Check sheet for the drawn part. Datum: minimum x, y, z corner. Units: mm. Round coordinates to 2 decimals unless told otherwise and drop trailing zeros. Write each loop counter-clockwise with the first axis right and the second up, starting at its lowest first coordinate (ties: lowest second). Pieces come first, ordered by that corner, then holes. Notation, with made-up numbers: (48, -9.75) - (106, -9.75) arc R24 ccw to (106, 0.25) - close; hole circle Ø8 at (-14, 12). An arc over 180 degrees is marked (long way). Answer as a JSON object with one key per item and string values. Group by question number.
Item 1: Sectioned sample at B-B on z = 164. Record the boundary of the cut face in (x, y).
Item 2: Thickness scan on line 1 (X direction, y = 0.85, z = 164); line 2 (Z direction, x = 65, y = 0.65) (3 decimals); line 3 (Z direction, x = 82, y = 1.25) (3 decimals). Record the ranges inside material, lowest first.
Item 3: Sectioned sample at A-A on x = 65. Record the boundary of the cut face in (y, z) (3 decimals).
Item 4: Gauge pin test, flat ends, axial feed: P1, Ø2.5, axis at x = 65, z = 164, coming from the +Y side; P2, Ø1.2, axis at y = 3, z = 2, coming from the +X side. Record the tip position at first contact, or that the pin passes through.
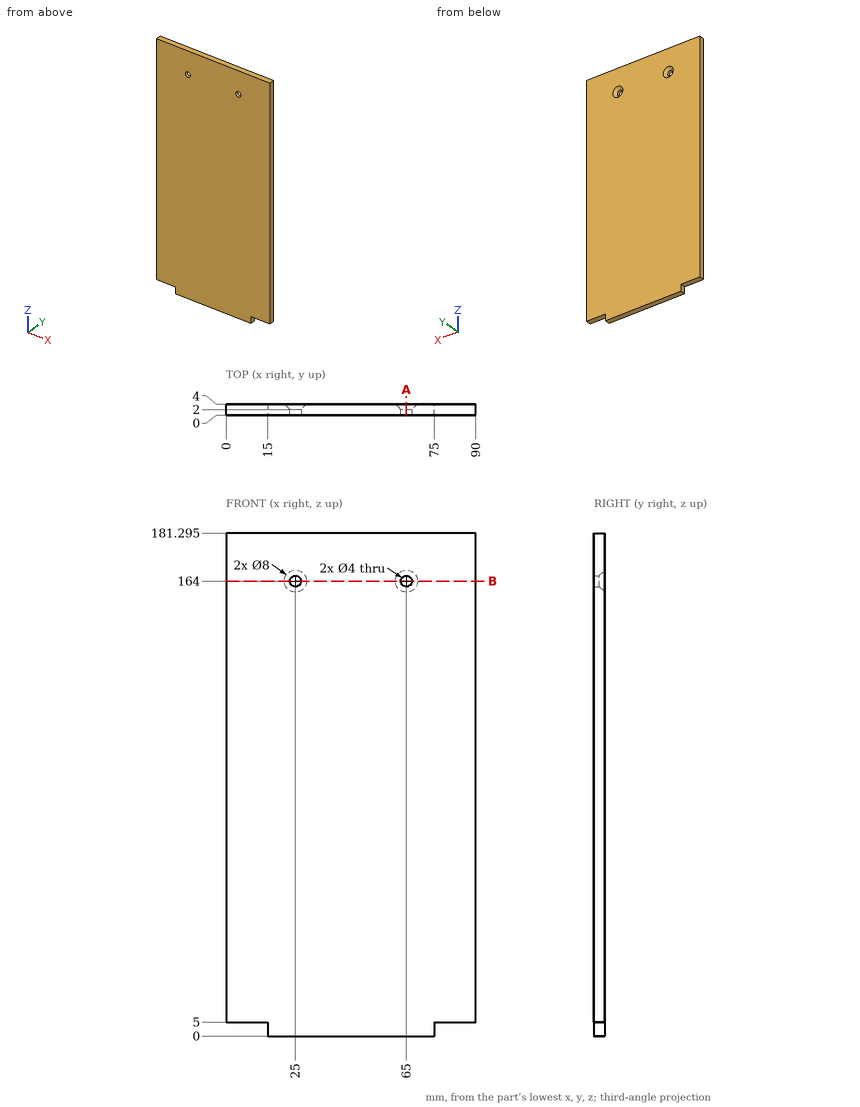
Completed:
{
 "1": {"outline": "(0, 0) - (23, 0) - (23, 2) - (21, 4) - (0, 4) - close; (27, 0) - (63, 0) - (63, 2) - (61, 4) - (29, 4) - (27, 2) - close; (67, 0) - (90, 0) - (90, 4) - (69, 4) - (67, 2) - close"},
 "2": {"line 1": "0 to 23, 27 to 63, 67 to 90", "line 2": "0 to 162, 166 to 181.295", "line 3": "5 to 181.295"},
 "3": {"outline": "(0, 0) - (4, 0) - (4, 160) - (2, 162) - (0, 162) - close; (0, 166) - (2, 166) - (4, 168) - (4, 181.295) - (0, 181.295) - close"},
 "4": {"P1": "through", "P2": "x = 75"}
}
